Build history of the part. All positions in model axes, mm. Face numbers are marked on the shaded views. A direction names the side the tool comes from. Give positions to 0.01 mm unless a question says otherwise; leave off trailing zeros. Write each loop counter-clockwise with the first axis right and the second up, starting at its lowest first coordinate (ties: lowest second). Pieces come first, ordered by that corner, then holes.
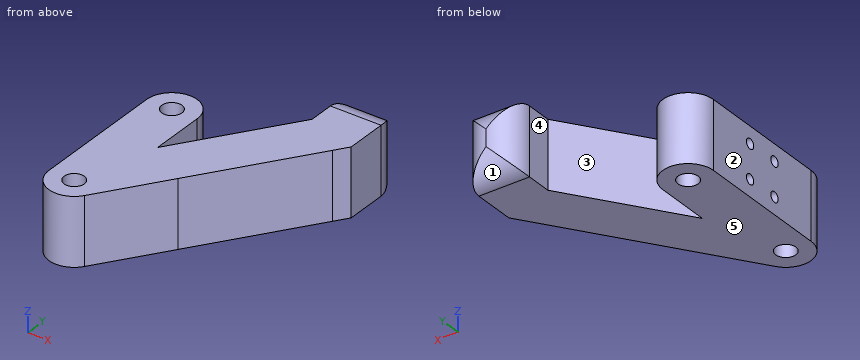
from build123d import *

# Parameters (mm, degrees)
SKETCH1_R           = 1.5
BOSS_EXTRUDE1_DEPTH = 10
FILLET1_R           = 3.75
SKETCH2_R           = 0.75
CUT_EXTRUDE1_DEPTH  = 7.5


with BuildPart() as part:
    # Sketch1 → Boss-Extrude1 (new body)
    with BuildSketch(Plane.XY):
        with BuildLine():
            Line((-3.75, 0), (-3.75, 20))
            ThreePointArc((-3.75, 20), (0, 23.75), (3.75, 20))
            Line((3.75, 20), (3.75, 11.893480509))
            Line((3.75, 11.893480509), (15, 27.960145585))
            Line((15, 27.960145585), (15, 35.460145585))
            Line((15, 35.460145585), (22.5, 35.460145585))
            Line((22.5, 35.460145585), (22.5, 25.595404668))
            Line((22.5, 25.595404668), (21.143640332, 23.658322312))
            Line((21.143640332, 23.658322312), (9.893640332, 7.591657236))
            Line((9.893640332, 7.591657236), (3.071820166, -2.150911636))
            ThreePointArc((3.071820166, -2.150911636), (-1.127646748, -3.576438565), (-3.75, 0))
        make_face()
        Circle(SKETCH1_R, mode=Mode.SUBTRACT)
        with Locations((0, 20)):
            Circle(SKETCH1_R, mode=Mode.SUBTRACT)
    extrude(amount=BOSS_EXTRUDE1_DEPTH)

    # Fillet1
    fillet1_edges = [part.edges().sort_by_distance(p)[0] for p in [
        (18.75, 35.460145585, 0),
        (22.5, 35.460145585, 5),
        (15, 35.460145585, 5),
        (18.75, 35.460145585, 10),
    ]]
    fillet(fillet1_edges, radius=FILLET1_R - 0.0001)  # a hair under: the kernel refuses the full size

    # Sketch2 → Cut-Extrude1 (cut)
    with BuildSketch(Plane.ZY.offset(3.75)):
        with Locations((7.5, 12.5)):
            Circle(SKETCH2_R)
        with Locations(Location((7.5, 7.5, 0), (0, 0, 180))):
            Circle(SKETCH2_R)
        with Locations((2.5, 7.5)):
            Circle(SKETCH2_R)
        with Locations(Location((2.5, 12.5, 0), (0, 0, 306.031603779))):
            Circle(SKETCH2_R)
    extrude(amount=-CUT_EXTRUDE1_DEPTH, mode=Mode.SUBTRACT)


solid = part.part
(1) Saw through at C-C, the plane z = 7.5. List the corners of the cut face in (x, y).
(2) Saw through at A-A, the plane x = 0. List the corners of the cut face in (y, z), plus the area to 3 significant figures.
(3) Drop flat-ended pins along their axis: pin 1 (2 mm diameter, centred on y = 12.5, z = 7.5, fed in from +X); pin 2 (3 mm diameter, centred on x = 17.5, z = 8, fed in from +Y); pin 3 (4 mm diameter, centred on y = 15, z = 4.5, fed in from +X); pin 4 (2.5 mm diameter, centred on x = 0, y = 0, fed in from +Z). Give the stop position or say it passes through.
(4) Probe line 1 (Y direction, x = 0, z = 7.5); line 2 (Z direction, x = 1.5, y = 12.5); line 3 (Y direction, x = 0, z = 3.75). List the from-to ranges inside material, lowest first.
(5) Saw through at D-D, the plane y = 22. List the corners of the cut face in (x, z), plus the area to 3 significant figures.
(6) Mould opens along X. For the marked faces 1, 2 and 3 say: +X half, -X half, draft (parallel to the pull), parting line (faces both ways), or undercut.
(7) Saw through at B-B, the plane z = 5.5. Give the number of separate pieces and of enclosed holes in the cut face, plus the area to 3 significant figures.
(8) 3-axis set-ups, long thin cutter, end or side, ignore diameter. For the marked faces 4 and 5: which of +Z, -Z, +X, -X, +Y, -Y reach the whole face in a straight line?
Computed values:
1. outline: (-3.75, 0) arc R3.75 ccw to (3.07, -2.15) - (22.5, 25.6) - (22.5, 31.71) arc R3.75 ccw to (20, 35.25) - (17.5, 35.25) arc R3.75 ccw to (15, 31.71) - (15, 27.96) - (3.75, 11.89) - (3.75, 11.75) - (-3.75, 11.75) - (-3.75, 8.25) - (3.75, 8.25) - (3.75, 6.75) - (-3.75, 6.75) - close; (-3.75, 13.25) - (3.75, 13.25) - (3.75, 20) arc R3.75 ccw to (-3.75, 20) - close; hole circle Ø3 at (0, 0); hole circle Ø3 at (0, 20)
2. outline: (-3.75, 0) - (-1.5, 0) - (-1.5, 10) - (-3.75, 10) - close; (1.5, 0) - (18.5, 0) - (18.5, 10) - (1.5, 10) - close; (21.5, 0) - (23.75, 0) - (23.75, 10) - (21.5, 10) - close; hole circle Ø1.5 at (7.5, 2.5); hole circle Ø1.5 at (7.5, 7.5); hole circle Ø1.5 at (12.5, 2.5); hole circle Ø1.5 at (12.5, 7.5)
2. area: 208 mm2
3. pin 1: stops at x = 14.03
3. pin 2: stops at y = 35.43
3. pin 3: stops at x = 16.48
3. pin 4: passes through
4. line 1: y = -3.75 to -1.5, 1.5 to 6.75, 8.25 to 11.75, 13.25 to 18.5, 21.5 to 23.75
4. line 2: z = 0 to 1.75, 3.25 to 6.75, 8.25 to 10
4. line 3: y = -3.75 to -1.5, 1.5 to 18.5, 21.5 to 23.75
5. outline: (-3.17, 0) - (3.17, 0) - (3.17, 10) - (-3.17, 10) - close; (10.83, 0) - (19.98, 0) - (19.98, 10) - (10.83, 10) - close
5. area: 155 mm2
6. face 1: draft
6. face 2: -X half
6. face 3: undercut
7. separate pieces: 1
7. enclosed holes: 2
7. area: 435 mm2
8. face 4: +Z, -Z, -X, +Y
8. face 5: -Z, +X, -X, +Y, -Y
